Drawing for the job (mm, zero at the part's lowest x, y, z). A direction names the side the tool comes from. Coordinates: 2 decimals unless noted, no trailing zeros. Loops run counter-clockwise (first coordinate to the right, second up) from the corner with the lowest first, then second, coordinate; pieces in that order, holes last. Notation, with made-up numbers: (-33, -24.75) - (20, -24.75) arc R16 cw to (20, 6.25) - close; hole circle Ø6 at (74, 8.25). An arc over 180 degrees is marked (long way). Put each result on its own line as item: value.
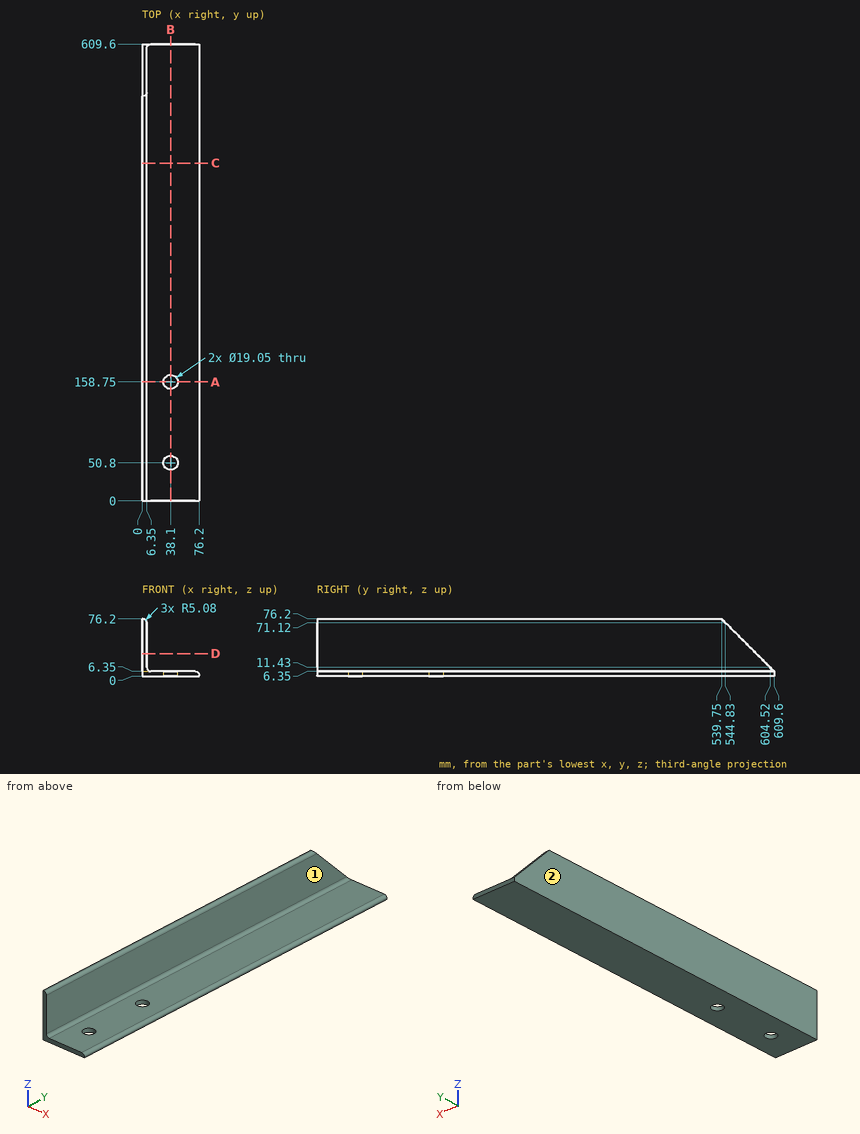
Q1. Slice it at C-C, the plane y = 450.5. Give the cut face in (x, z), then the cut area to 3 significant figures.
Determined:
outline: (0, 0) - (76.2, 0) - (76.2, 1.27) arc R5.08 ccw to (71.12, 6.35) - (11.43, 6.35) arc R5.08 cw to (6.35, 11.43) - (6.35, 71.12) arc R5.08 ccw to (1.27, 76.2) - (0, 76.2) - close
area: 922 mm2
Q2. Slice it at A-A, the plane y = 158.75. Give the cut face in (x, z) (3 decimals), then the cut area to 3 significant figures.
Determined:
outline: (0, 0) - (28.575, 0) - (28.575, 6.35) - (11.43, 6.35) arc R5.08 cw to (6.35, 11.43) - (6.35, 71.12) arc R5.08 ccw to (1.27, 76.2) - (0, 76.2) - close; (47.625, 0) - (76.2, 0) - (76.2, 1.27) arc R5.08 ccw to (71.12, 6.35) - (47.625, 6.35) - close
area: 801 mm2
Q3. Wall check: L1, parallel to Y at x = 38, z = 3; L2, parallel to X at y = 158.75, z = 2 (3 decimals); L3, parallel to X at y = 180, z = 67. Give the ranges that are in metal, low to high. Write a range as from..to.
Determined:
L1: 0..41.28, 60.32..149.23, 168.27..609.6
L2: 0..28.575, 47.625..76.147
L3: 0..6.35
Q4. Pin check, flat tips, straight feed: pin 1 Ø6 at (x, y) = (62.5, 236.5) entering from +Z; pin 2 Ø10 at (y, z) = (213, 64) entering from +X; pin 3 Ø2 at (y, z) = (210.5, 55) entering from +X. Stop position of each tip, or through.
Determined:
pin 1: z = 6.35
pin 2: x = 6.35
pin 3: x = 6.35
Q5. Tool access for the marked faces 1 and 2: list every direction of +Z, -Z, +X, -X, +Y, -Y with a clear straight run to the whole face (end or side of a thin tool).
Determined:
face 1: +Z, +X, +Y, -Y
face 2: +Z, -Z, -X, +Y, -Y
Q6. Slice it at D-D, the plane z = 30. Give the cut face in (x, y), then the cut area to 3 significant figures.
Determined:
outline: (0, 0) - (6.35, 0) - (6.35, 585.95) - (0, 585.95) - close
area: 3,720 mm2
Q7. Slice it at B-B, the plane x = 38.1. Give the cut face in (y, z) (3 decimals).
Determined:
outline: (0, 0) - (41.275, 0) - (41.275, 6.35) - (0, 6.35) - close; (60.325, 0) - (149.225, 0) - (149.225, 6.35) - (60.325, 6.35) - close; (168.275, 0) - (609.6, 0) - (609.6, 6.35) - (168.275, 6.35) - close
